CAD build for the part. Positions are in the model's coordinates, mm. A direction names the side the tool comes from. Round coordinates to 2 decimals unless told otherwise and drop trailing zeros. Write each loop counter-clockwise with the first axis right and the second up, starting at its lowest first coordinate (ties: lowest second). Pieces come first, ordered by that corner, then holes. Notation, with made-up numbers: (-37, -17.75) - (-1, -17.75) arc R27 cw to (-1, 7.25) - close; hole circle Ø6 at (-30.75, 20). An arc over 180 degrees is marked (long way). Answer in a Markdown table with one row per item.
```python
from build123d import *

# Parameters (mm, degrees)
EXTRUDE_1_DEPTH        = 14.4
CUT_EXTRUDE_1_REACH    = 4
EXTRUDE_2_DEPTH        = 1.5
SKETCH_4_W             = 6.8
SKETCH_4_H             = 3.6
EXTRUDE_3_DEPTH        = 7.8
SKETCH_5_W             = 19
SKETCH_5_H             = 2.1
EXTRUDE_4_DEPTH        = 7.8
EXTRUDE_5_DEPTH        = 1.5
HOLE_WIZARD_M3_1_D     = 2.5
HOLE_WIZARD_M3_1_DEPTH = 6.5
HOLE_WIZARD_M3_1_TIP   = 0.751075774
FILLET_1_R             = 0.5
FILLET_2_R             = 1


with BuildPart() as part:
    # 草图1 → 凸台-拉伸1 (new body)
    with BuildSketch(Plane.XY):
        with BuildLine():
            Line((16, 0), (-16, 0))
            ThreePointArc((-16, 0), (-20.949747468, 2.050252532), (-23, 7))
            Line((-23, 7), (-23, 9.4))
            ThreePointArc((-23, 9.4), (-22.824264069, 9.824264069), (-22.4, 10))
            Line((-22.4, 10), (-22.179247695, 10))
            ThreePointArc((-22.179247695, 10), (-21.743961945, 9.812948321), (-21.580079296, 9.368421053))
            ThreePointArc((-21.580079296, 9.368421053), (-19.668115061, 4.182269589), (-14.58978131, 2))
            Line((-14.58978131, 2), (14.58978131, 2))
            ThreePointArc((14.58978131, 2), (19.668115061, 4.182269589), (21.580079296, 9.368421053))
            ThreePointArc((21.580079296, 9.368421053), (21.743961945, 9.812948321), (22.179247695, 10))
            Line((22.179247695, 10), (22.4, 10))
            ThreePointArc((22.4, 10), (22.824264069, 9.824264069), (23, 9.4))
            Line((23, 9.4), (23, 7))
            ThreePointArc((23, 7), (20.949747468, 2.050252532), (16, 0))
        make_face()
    extrude(amount=EXTRUDE_1_DEPTH)

    # 草图2 → 切除-拉伸1 (cut, up to next)
    with BuildSketch(Plane(origin=(0, 2, 0), x_dir=(1, 0, 0), z_dir=(0, 1, 0)), mode=Mode.PRIVATE) as cut_extrude_1_sk1:
        Polygon((4, -2.2), (-4, -2.2), (-6.2, 0), (6.2, 0), align=None)
    cut_extrude_1_tool1 = extrude(cut_extrude_1_sk1.sketch, amount=-CUT_EXTRUDE_1_REACH, mode=Mode.PRIVATE) & part.part
    add(cut_extrude_1_tool1.solids().sort_by_distance((0, 2, 1.020915))[0], mode=Mode.SUBTRACT)

    # 草图3 → 凸台-拉伸2 (add)
    with BuildSketch(Plane.XY):
        Polygon((-7.75, 2), (-7.75, -7.8), (-14.55, -7.8), (-23, 3.2), (-23, 8.2), (-22.047090089, 8.2), (-19.556592195, 2.646086111), (-16.835492645, 2), align=None)
        Polygon((16.835492645, 2), (7.75, 2), (7.75, -7.8), (14.55, -7.8), (23, 3.2), (23, 8.2), (22.047090089, 8.2), (19.556592195, 2.646086111), align=None)
    extrude(amount=EXTRUDE_2_DEPTH)

    # 草图4 → 凸台-拉伸3 (add)
    with BuildSketch(Plane.XZ):
        with Locations((-11.15, 3.3)):
            Rectangle(SKETCH_4_W, SKETCH_4_H)
        with Locations((11.15, 3.3)):
            Rectangle(SKETCH_4_W, SKETCH_4_H)
    extrude(amount=EXTRUDE_3_DEPTH)

    # 草图5 → 凸台-拉伸4 (add)
    with BuildSketch(Plane.XZ):
        with Locations((0, 14.35)):
            Rectangle(SKETCH_5_W, SKETCH_5_H)
    extrude(amount=EXTRUDE_4_DEPTH)

    # 草图6 → 凸台-拉伸5 (add)
    with BuildSketch(Plane.XY.offset(14.4)):
        Polygon((-7.75, 0), (-20.541818182, 0), (-23, 3.2), (-23, 8.2), (-22.047090089, 8.2), (-19.556592195, 2.646086111), (-16.835492645, 2), (-7.75, 2), align=None)
        Polygon((7.75, 0), (20.541818182, 0), (23, 3.2), (23, 8.2), (22.047090089, 8.2), (19.556592195, 2.646086111), (16.835492645, 2), (7.75, 2), align=None)
    extrude(amount=-EXTRUDE_5_DEPTH)

    # M3 螺纹孔1
    with Locations(Plane(origin=(0, -7.8, 0), x_dir=(-1, 0, 0), z_dir=(0, -1, 0))):
        with Locations((-11.15, -2.55), (11.15, -2.55)):
            Hole(HOLE_WIZARD_M3_1_D / 2, depth=HOLE_WIZARD_M3_1_DEPTH)
            with Locations((0, 0, -(HOLE_WIZARD_M3_1_DEPTH + HOLE_WIZARD_M3_1_TIP / 2))):  # 118° drill point
                Cone(0, HOLE_WIZARD_M3_1_D / 2, HOLE_WIZARD_M3_1_TIP, mode=Mode.SUBTRACT)

    # 圆角1
    fillet_1_edges = [part.edges().sort_by_distance(p)[0] for p in [
        (9.5, -7.8, 14.35),
        (-9.5, -7.8, 14.35),
        (-20.541818182, 0, 13.65),
        (-23, 3.2, 13.65),
        (20.541818182, 0, 13.65),
        (23, 3.2, 13.65),
        (-23, 3.2, 0.75),
        (23, 3.2, 0.75),
    ]]
    fillet(fillet_1_edges, radius=FILLET_1_R)

    # 圆角2
    fillet_2_edges = [part.edges().sort_by_distance(p)[0] for p in [
        (-6.2, 1, 0),
        (6.2, 1, 0),
        (4, 1, 2.2),
        (-4, 1, 2.2),
    ]]
    fillet(fillet_2_edges, radius=FILLET_2_R)


solid = part.part
```
Q1. Saw through at D-D on z = 4.25. List the corners of the cut face in (x, y).
Computed:
| item | result |
|---|---|
| outline | (-23, 7) arc R7 ccw to (-16, 0) - (-14.55, 0) - (-14.55, -7.8) - (-7.75, -7.8) - (-7.75, 0) - (7.75, 0) - (7.75, -7.8) - (14.55, -7.8) - (14.55, 0) - (16, 0) arc R7 ccw to (23, 7) - (23, 9.4) arc R0.6 ccw to (22.4, 10) - (22.18, 10) arc R0.6 ccw to (21.58, 9.37) arc R7 cw to (14.59, 2) - (-14.59, 2) arc R7 cw to (-21.58, 9.37) arc R0.6 ccw to (-22.18, 10) - (-22.4, 10) arc R0.6 ccw to (-23, 9.4) - close |
Q2. Saw through at B-B on x = 1.5. List the corners of the cut face in (y, z).
Computed:
| item | result |
|---|---|
| outline | (-7.8, 13.3) - (0, 13.3) - (0, 2.2) - (2, 2.2) - (2, 14.4) - (0, 14.4) - (0, 15.4) - (-7.8, 15.4) - close |
Q3. Drill centre lines: line 1 (Z direction, x = 11.15, y = -2.25); line 2 (Z direction, x = -8.5, y = -6.5); line 3 (X direction, y = 8.5, z = 6.5). Where is each one in solid material? Low to high.
Computed:
| item | result |
|---|---|
| line 1 | z = 0 to 1.3, 3.8 to 5.1 |
| line 2 | z = 0 to 5.1, 13.3 to 15.4 |
| line 3 | x = -23 to -21.57, 21.57 to 23 |
Q4. Pull direction X, two halves, no side cores. Call faces 4 (the flat face through (9.5, -4, 14)), 5 (the flat face through (0.1, 1.7, 14.4)), 6 (the flat face through (-18.7, -2.4, 0.7)), 7 (the flat face through (-7.75, -4, 3)): released by +X, released by -X, zero draft, split by the parting line, or undercut.
Computed:
| item | result |
|---|---|
| face 4 | released by +X |
| face 5 | zero draft |
| face 6 | released by -X |
| face 7 | undercut |
Q5. 3-axis set-ups, long thin cutter, end or side, ignore diameter. For faces 1 (the flat face through (0, 2, 7)), 2 (the flat face through (-18, -1, 1.5)), 3 (the flat face through (0, 1, 2.2)): which of +Z, -Z, +X, -X, +Y, -Y reach the whole face in a straight line?
Computed:
| item | result |
|---|---|
| face 1 | +Z, -Z, +Y |
| face 2 | -X, -Y |
| face 3 | -Z, +Y, -Y |
Q6. Saw through at C-C on y = 5.25. List the corners of the cut face in (x, z), then the cut area to 3 significant figures.
Computed:
| item | result |
|---|---|
| outline | (-23, 0) - (-20.5, 0) - (-20.5, 14.4) - (-23, 14.4) - (-23, 12.9) - (-22.78, 12.9) - (-22.78, 1.5) - (-23, 1.5) - close; (20.5, 0) - (23, 0) - (23, 1.5) - (22.78, 1.5) - (22.78, 12.9) - (23, 12.9) - (23, 14.4) - (20.5, 14.4) - close |
| area | 66.9 mm2 |
Q7. Saw through at A-A on y = -2. List the corners of the cut face in (x, z).
Computed:
| item | result |
|---|---|
| outline | (-19.01, 0) - (-7.75, 0) - (-7.75, 5.1) - (-14.55, 5.1) - (-14.55, 1.5) - (-19.01, 1.5) - close; (-9.5, 13.3) - (9.5, 13.3) - (9.5, 15.4) - (-9.5, 15.4) - close; (7.75, 0) - (19.01, 0) - (19.01, 1.5) - (14.55, 1.5) - (14.55, 5.1) - (7.75, 5.1) - close; hole circle Ø2.5 at (-11.15, 2.55); hole circle Ø2.5 at (11.15, 2.55) |
Q8. Flat gauge pins, fed straight in: pin 1 (3.5 mm diameter, centred on x = 20, y = 3.5, fed in from -Z); pin 2 (3 mm diameter, centred on x = -13, y = 2.5, fed in from +Z); pin 3 (1.1 mm diameter, centred on y = -2, z = 3, fed in from +X); pin 4 (6 mm diameter, centred on x = 3.5, y = -5.5, fed in from -Z). Where does each tip first touch, or does it go through?
Computed:
| item | result |
|---|---|
| pin 1 | stops at z = 0 |
| pin 2 | stops at z = 14.4 |
| pin 3 | stops at x = 14.55 |
| pin 4 | stops at z = 13.3 |
